```python
from build123d import *

# Parameters (mm, degrees)
F0_R     = 57.15
F0_R_2   = 50.8
F1_DEPTH = 25.4
F0_R_3   = 38.1
F2_DEPTH = 31.75
F0_R_4   = 3.175
F3_DEPTH = 19.05


with BuildPart() as f1:
    # F0 (on Front) → F1 (new body)
    with BuildSketch(Plane.XZ):
        Circle(F0_R)
        Circle(F0_R_2, mode=Mode.SUBTRACT)
    extrude(amount=F1_DEPTH)

    # F0 (on Front) → F2 (join)
    with BuildSketch(Plane.XZ):
        Circle(F0_R_2)
        Circle(F0_R_3, mode=Mode.SUBTRACT)
    extrude(amount=F2_DEPTH)

    # F0 (on Front) → F3 (join)
    with BuildSketch(Plane.XZ):
        Circle(F0_R_3)
        with Locations((-17.960512, -17.960512)):
            Circle(F0_R_4, mode=Mode.SUBTRACT)
        with Locations((0, -25.4)):
            Circle(F0_R_4, mode=Mode.SUBTRACT)
        with Locations((17.960512, -17.960512)):
            Circle(F0_R_4, mode=Mode.SUBTRACT)
        with Locations((-25.4, 0)):
            Circle(F0_R_4, mode=Mode.SUBTRACT)
        with Locations((-17.960512, 17.960512)):
            Circle(F0_R_4, mode=Mode.SUBTRACT)
        Circle(F0_R_4, mode=Mode.SUBTRACT)
        with Locations((25.4, 0)):
            Circle(F0_R_4, mode=Mode.SUBTRACT)
        with Locations((0, 25.4)):
            Circle(F0_R_4, mode=Mode.SUBTRACT)
        with Locations((17.960512, 17.960512)):
            Circle(F0_R_4, mode=Mode.SUBTRACT)
    extrude(amount=F3_DEPTH)


solid = f1.part
```
Input: part model. Units: mm. Frame: model coordinates. A direction names the side the tool comes from. Coordinates: 2 decimals unless noted, no trailing zeros. Loops run counter-clockwise (first coordinate to the right, second up) from the corner with the lowest first, then second, coordinate; pieces in that order, holes last. Notation, with made-up numbers: M 78.25,43 L 88.25,43 A18 ccw 88.25,78 Z; hole C 64,68 d8. An arc over 180 degrees is marked long. One line per item, written item: value.
(1) Pull-direction query (Z, two-part tool) for faces 3 (the flat face through (-1, 0, -12)), 4 (the cylindrical face through (-57.095, -12.522, 2.513)), 5 (the cylindrical face through (-0.69, -9.39, -3.1)); classes: +Z half, -Z half, draft (parallel to the pull), parting line (faces both ways), or undercut.
Filled in:
face 3: draft
face 4: parting line
face 5: undercut
(2) Pin query (flat end, axial travel): pin 1 (1.5 mm diameter, centred on x = 43, z = -18, fed in from +Y); pin 2 (5 mm diameter, centred on x = -17.96, z = 17.96, fed in from +Y); pin 3 (10 mm diameter, centred on x = 13.5, y = -12.5, fed in from +Z); pin 4 (1.5 mm diameter, centred on x = -5, z = -17, fed in from -Y). Return the tip coordinate at first contact, or that it passes through.
Filled in:
pin 1: y = 0
pin 2: through
pin 3: z = 56.51
pin 4: y = -19.05
(3) Line query: line 1 along Z through (x, y) = (0, -7) (3 decimals); line 2 along Z through (x, y) = (19.5, -6); line 3 along Y through (x, z) = (6.5, -8.5). Output: solid intervals per line, ascending. Write a range as from..to.
Filled in:
line 1: -57.15..-28.575, -22.225..-3.175, 3.175..22.225, 28.575..57.15
line 2: -53.72..-20.74, -15.18..15.18, 20.74..53.72
line 3: -19.05..0
(4) Section C-C (z = 25.4). Output: boundary loops of the cut face in (x, y) (3 decimals), and give its area (3 significant figures).
Filled in:
outline: M -51.195,-25.4 L -43.994,-25.4 L -43.994,-31.75 L -28.398,-31.75 L -28.398,-19.05 L -3.175,-19.05 L -3.175,0 L -51.195,0 Z; M 3.175,-19.05 L 28.398,-19.05 L 28.398,-31.75 L 43.994,-31.75 L 43.994,-25.4 L 51.195,-25.4 L 51.195,0 L 3.175,0 Z
area: 2,320 mm^2
(5) Reachability of faces 1 (the cylindrical face through (28.43, -9.39, 0.95)), 2 (the cylindrical face through (-11.012, -28.531, -49.592)) from +Z, -Z, +X, -X, +Y, -Y: full face, straight path, thin tool, end or side. Return the list, or none.
Filled in:
face 1: +Y, -Y
face 2: -Y
(6) Section A-A (x = 24). Output: boundary loops of the cut face in (y, z), and give its area (3 significant figures).
Filled in:
outline: M -31.75,-44.77 L -25.4,-44.77 L -25.4,-51.87 L 0,-51.87 L 0,-2.85 L -19.05,-2.85 L -19.05,-29.59 L -31.75,-29.59 Z; M -31.75,29.59 L -19.05,29.59 L -19.05,2.85 L 0,2.85 L 0,51.87 L -25.4,51.87 L -25.4,44.77 L -31.75,44.77 Z
area: 2,340 mm^2
(7) Section D-D (y = -10). Give the number of separate pieces and of enclosed holes in the cut face, and give its area (3 significant figures).
Filled in:
separate pieces: 1
enclosed holes: 9
area: 9,980 mm^2
(8) Section B-B (x = 0). Output: boundary loops of the cut face in (y, z) (3 decimals), and give its area (3 significant figures).
Filled in:
outline: M -31.75,-50.8 L -25.4,-50.8 L -25.4,-57.15 L 0,-57.15 L 0,-28.575 L -19.05,-28.575 L -19.05,-38.1 L -31.75,-38.1 Z; M -31.75,38.1 L -19.05,38.1 L -19.05,28.575 L 0,28.575 L 0,57.15 L -25.4,57.15 L -25.4,50.8 L -31.75,50.8 Z; M -19.05,-22.225 L 0,-22.225 L 0,-3.175 L -19.05,-3.175 Z; M -19.05,3.175 L 0,3.175 L 0,22.225 L -19.05,22.225 Z
area: 2,220 mm^2
